Geometry check sheet. Reference: the model listing, model coordinates, mm. Give positions to 0.01 mm unless a question says otherwise; leave off trailing zeros. Write each loop counter-clockwise with the first axis right and the second up, starting at its lowest first coordinate (ties: lowest second). Pieces come first, ordered by that corner, then holes. Notation, with made-up numbers: (32.25, -7.5) -> (75.25, -7.5) arc R18 ccw to (75.25, 26.5) -> close; hole circle Ø11 at (-12.75, 17). An arc over 180 degrees is marked (long way). One line per item, written item: value.
Autodesk Inventor part; units mm, degrees
ref_plane "YZ Plane" through (0, 0, 0) normal (1, 0, 0) x (0, 1, 0)
ref_plane "XZ Plane" through (0, 0, 0) normal (0, 1, 0) x (-1, 0, 0)
ref_plane "XY Plane" through (0, 0, 0) normal (0, 0, 1) x (1, 0, 0)
sketch "Sketch1" plane through (0, 0, 0) normal (0, 1, 0) x (-1, 0, 0)
  line L0 (21, -25) -> (18.25, -25)
  line L1 (21, -48) -> (18.25, -48)
  line L2 (21, -143) -> (18.25, -143)
  line L3 (21, -68) -> (18.25, -68)
  line L4 (21, -128) -> (18.25, -128)
  line L5 (21, -108) -> (18.25, -108)
  line L6 (2.75, -68) -> (0, -68)
  line L7 (2.75, -108) -> (0, -108)
  line L8 (2.75, -128) -> (0, -128)
  line L9 (2.75, -143) -> (0, -143)
  line L10 (2.75, -48) -> (0, -48)
  line L11 (2.75, -25) -> (0, -25)
  line L12 (21, -158) -> (21, -143)
  line L13 (21, -128) -> (21, -108)
  line L14 (21, -68) -> (21, -48)
  line L15 (21, -25) -> (21, 0)
  line L16 (0, -158) -> (0, -143)
  line L17 (0, -128) -> (0, -108)
  line L18 (0, -68) -> (0, -48)
  line L19 (0, -25) -> (0, 0)
  line L20 (18.25, -143) -> (18.25, -128)
  line L21 (18.25, -108) -> (18.25, -68)
  line L22 (18.25, -48) -> (18.25, -25)
  line L23 (2.75, -143) -> (2.75, -128)
  line L24 (2.75, -108) -> (2.75, -68)
  line L25 (2.75, -48) -> (2.75, -25)
  line L26 (21, -68) -> (21, -48) construction
  line L27 (10.5, -68) -> (10.5, -97) construction
  line L28 (18.25, -158) -> (18.25, -178)
  line L29 (18.25, -178) -> (21, -178)
  line L30 (21, -178) -> (21, -196)
  line L31 (0, -196) -> (0, -178)
  line L32 (0, -178) -> (2.75, -178)
  line L33 (2.75, -158) -> (2.75, -178)
  line L34 (21, -158) -> (18.25, -158)
  line L35 (2.75, -158) -> (0, -158)
  line L36 (7.55, -176) -> (5.75, -176)
  line L37 (5.75, -176) -> (5.75, -186)
  line L38 (5.75, -186) -> (7.55, -186)
  line L39 (7.55, -186) -> (7.55, -176)
  line L40 (18.25, 0) -> (18.25, 2.75)
  line L41 (18.25, 2.75) -> (2.75, 2.75)
  line L42 (2.75, 2.75) -> (2.75, 0)
  line L43 (21, 0) -> (18.25, 0)
  line L44 (2.75, 0) -> (0, 0)
  line L45 (18.25, -196) -> (18.25, -198.75)
  line L46 (18.25, -198.75) -> (2.75, -198.75)
  line L47 (2.75, -198.75) -> (2.75, -196)
  line L48 (21, -196) -> (18.25, -196)
  line L49 (2.75, -196) -> (0, -196)
  line L50 (14, 0) -> (7, 0)
  line L51 (7, 0) -> (7, -3)
  line L52 (7, -3) -> (14, -3)
  line L53 (14, -3) -> (14, 0)
  line L54 (14, -193) -> (7, -193)
  line L55 (7, -193) -> (7, -196)
  line L56 (7, -196) -> (14, -196)
  line L57 (14, -196) -> (14, -193)
  dimension "d7" = 23
  dimension "d8" = 20
  dimension "d9" = 40
  dimension "d10" = 20
  dimension "d11" = 15
  dimension "d28" = 15.5
  dimension "d31" = 2.75
  dimension "d44" = 18
  dimension "d45" = 20
  dimension "d47" = 15
  dimension "d49" = 1.8
  dimension "d51" = 10
  dimension "d53" = 3
  dimension "d55" = 25
  dimension "d56" = 10
  dimension "d57" = 7
  dimension "d58" = 3
extrude "Extrusion3" add sketch "Sketch1" along normal blind 3
properties part number "Right_wall"
1) Sectioned sample at B-B on y = 0.65. Give the number of separate pieces and of enclosed holes in the cut face, plus the area to 3 significant figures.
Verdict:
separate pieces: 1
enclosed holes: 3
area: 3,600 mm^2
2) Sectioned sample at C-C on z = -137. Record the cut outline in (x, y), plus the area to 3 significant figures.
Verdict:
outline: (-18.25, 0) -> (-2.75, 0) -> (-2.75, 3) -> (-18.25, 3) -> close
area: 46.5 mm^2
3) Sectioned sample at A-A on z = -182. Record the cut outline in (x, y).
Verdict:
outline: (-21, 0) -> (-7.55, 0) -> (-7.55, 3) -> (-21, 3) -> close; (-5.75, 0) -> (0, 0) -> (0, 3) -> (-5.75, 3) -> close
4) Depth check by flat-ended pin: pin 1 Ø1.4 at (y, z) = (1.5, 1) entering from +X; pin 2 Ø1.4 at (x, y) = (-1.5, 1) entering from +Z; pin 3 Ø10 at (x, z) = (-8, -71.5) entering from -Y; pin 4 Ø1.4 at (x, y) = (-2, 1) entering from -Z. Enter the tip coordinate at first touch or a pass-through.
Verdict:
pin 1: x = -2.75
pin 2: z = 0
pin 3: y = 0
pin 4: z = -196
5) Scan lines: probe 1 along Z at (x, y) = (-8, 0.3); probe 2 along Z at (x, y) = (-7.5, 1.9); probe 3 along X at (y, z) = (1.85, -76). Record each from-to range of solid material in increasing order.
Verdict:
probe 1: -198.75 to -196, -193 to -3, 0 to 2.75
probe 2: -198.75 to -196, -193 to -186, -176 to -3, 0 to 2.75
probe 3: -18.25 to -2.75
